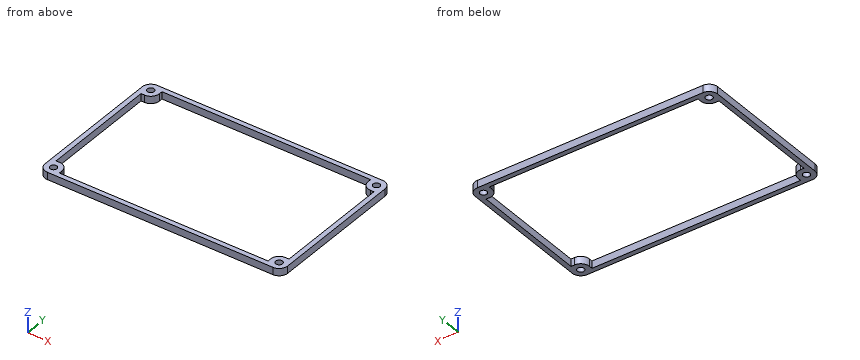
```python
from build123d import *

# Parameters (mm, degrees)
SKETCH1_R           = 1.4
BOSS_EXTRUDE1_DEPTH = 3
SKETCH2_W           = 5
SKETCH2_H           = 48
SKETCH2_W_2         = 86
SKETCH2_H_2         = 5
CUT_EXTRUDE1_DEPTH  = 3
FILLET1_R           = 3.5


with BuildPart() as part:
    # Sketch1 → Boss-Extrude1 (new body)
    with BuildSketch(Plane.XY):
        with BuildLine():
            Line((-46.5, -31), (46.5, -31))
            ThreePointArc((46.5, -31), (48.974873734, -29.974873734), (50, -27.5))
            Line((50, -27.5), (50, 27.5))
            ThreePointArc((50, 27.5), (48.974873734, 29.974873734), (46.5, 31))
            Line((46.5, 31), (-46.5, 31))
            ThreePointArc((-46.5, 31), (-48.974873734, 29.974873734), (-50, 27.5))
            Line((-50, 27.5), (-50, -27.5))
            ThreePointArc((-50, -27.5), (-48.974873734, -29.974873734), (-46.5, -31))
        make_face()
        with Locations((-46.5, 27.5)):
            Circle(SKETCH1_R, mode=Mode.SUBTRACT)
        with Locations((46.5, 27.5)):
            Circle(SKETCH1_R, mode=Mode.SUBTRACT)
        with Locations((46.5, -27.5)):
            Circle(SKETCH1_R, mode=Mode.SUBTRACT)
        with Locations((-46.5, -27.5)):
            Circle(SKETCH1_R, mode=Mode.SUBTRACT)
    extrude(amount=BOSS_EXTRUDE1_DEPTH)

    # Sketch2 → Cut-Extrude1 (cut)
    with BuildSketch(Plane.XY.offset(3)):
        with Locations((-45.5, 0)):
            Rectangle(SKETCH2_W, SKETCH2_H)
        Rectangle(SKETCH2_W_2, SKETCH2_H)
        with Locations((0, 26.5)):
            Rectangle(SKETCH2_W_2, SKETCH2_H_2)
        with Locations((45.5, 0)):
            Rectangle(SKETCH2_W, SKETCH2_H)
        with Locations((0, -26.5)):
            Rectangle(SKETCH2_W_2, SKETCH2_H_2)
    extrude(amount=-CUT_EXTRUDE1_DEPTH, mode=Mode.SUBTRACT)

    # Fillet1
    fillet1_edges = [part.edges().sort_by_distance(p)[0] for p in [
        (-43, 24, 1.5),
        (43, 24, 1.5),
        (43, -24, 1.5),
        (-43, -24, 1.5),
    ]]
    fillet(fillet1_edges, radius=FILLET1_R)


solid = part.part
```
Geometry check sheet. Reference: the model listing, model coordinates, mm. Round coordinates to 2 decimals unless told otherwise and drop trailing zeros. Order: outer loops, then holes, each group sorted by start corner. A loop starts at its lowest first (then second) coordinate and runs counter-clockwise, first axis right, second up. Notation, with made-up numbers: M -1.5,42 L 6.5,42 A21 cw 6.5,74 Z; hole C 14.5,-7 d2. An arc over 180 degrees is marked long. Write item = value, one per line.
Q1. Depth check by flat-ended pin: pin 1 Ø0.8 at (y, z) = (28, 1) entering from -X; pin 2 Ø2 at (x, y) = (46.5, -27.5) entering from +Z; pin 3 Ø0.8 at (x, z) = (-47.5, 1.5) entering from -Y. Enter the tip coordinate at first touch or a pass-through.
Answer block:
pin_1 = -50
pin_2 = through
pin_3 = -30.95
Q2. Section check C-C (x = 9.5). Enter the section's corners in (y, z).
Answer block:
outline = M -31,0 L -29,0 L -29,3 L -31,3 Z; M 29,0 L 31,0 L 31,3 L 29,3 Z
Q3. Section check A-A (y = -13). Enter the section's corners in (x, z), plus the area to 3 significant figures.
Answer block:
outline = M -50,0 L -48,0 L -48,3 L -50,3 Z; M 48,0 L 50,0 L 50,3 L 48,3 Z
area = 12.0 mm^2
Q4. Scan lines: line 1 (Y direction, x = 46.5, z = 0.8); line 2 (X direction, y = -23, z = 2.95); line 3 (Y direction, x = 39.5, z = 1). Record each from-to range of solid material in increasing order.
Answer block:
line_1 = -31 to -28.9, -26.1 to -24, 24 to 26.1, 28.9 to 31
line_2 = -50 to -48, 48 to 50
line_3 = -31 to -29, 29 to 31
Q5. Section check B-B (z = 1.85). Enter the section's corners in (x, y), plus the area to 3 significant figures.
Answer block:
outline = M -50,-27.5 A3.5 ccw -46.5,-31 L 46.5,-31 A3.5 ccw 50,-27.5 L 50,27.5 A3.5 ccw 46.5,31 L -46.5,31 A3.5 ccw -50,27.5 Z; hole M -48,-24 L -46.5,-24 A3.5 cw -43,-27.5 L -43,-29 L 43,-29 L 43,-27.5 A3.5 cw 46.5,-24 L 48,-24 L 48,24 L 46.5,24 A3.5 cw 43,27.5 L 43,29 L -43,29 L -43,27.5 A3.5 cw -46.5,24 L -48,24 Z; hole C -46.5,-27.5 d2.8; hole C -46.5,27.5 d2.8; hole C 46.5,-27.5 d2.8; hole C 46.5,27.5 d2.8
area = 686 mm^2
